from build123d import *

# Parameters (mm, degrees)
SKETCH1_R           = 3.29
BOSS_EXTRUDE1_DEPTH = 22
SKETCH2_W           = 24
SKETCH2_H           = 11
BOSS_EXTRUDE2_DEPTH = 3
SKETCH3_W           = 12
SKETCH3_H           = 25
CUT_EXTRUDE1_DEPTH  = 20.25


with BuildPart() as part:
    # Sketch1 → Boss-Extrude1 (new body)
    with BuildSketch(Plane(origin=(0, 0, 0), x_dir=(1, 0, 0), z_dir=(0, 1, 0))):
        Polygon((24, -29), (-24, -29), (-31, -21.49418526), (-32, 21.49418526), (-25, 29), (25, 29), (32, 21.49418526), (31, -21.49418526), align=None)
        with Locations(Location((-26.933648737, -2.8, 0), (0, 0, 270))):
            Circle(SKETCH1_R, mode=Mode.SUBTRACT)
        with Locations(Location((26.933648737, -2.8, 0), (0, 0, 270))):
            Circle(SKETCH1_R, mode=Mode.SUBTRACT)
    extrude(amount=BOSS_EXTRUDE1_DEPTH)

    # Sketch2 → Boss-Extrude2 (add)
    with BuildSketch(Plane.XY.offset(29)):
        with Locations((0, 5.5)):
            Rectangle(SKETCH2_W, SKETCH2_H)
    extrude(amount=BOSS_EXTRUDE2_DEPTH)

    # Sketch3 → Cut-Extrude1 (cut)
    with BuildSketch(Plane(origin=(0, 22, 0), x_dir=(1, 0, 0), z_dir=(0, 1, 0))):
        with Locations((-25.783797684, -0.3)):
            Rectangle(SKETCH3_W, SKETCH3_H)
        with Locations((25.783797684, -0.3)):
            Rectangle(SKETCH3_W, SKETCH3_H)
    extrude(amount=-CUT_EXTRUDE1_DEPTH, mode=Mode.SUBTRACT)


solid = part.part
For this review, take the finished solid that the model builds, in its own axes (mm). A direction names the side the tool comes from. Round coordinates to 2 decimals unless told otherwise and drop trailing zeros. Write each loop counter-clockwise with the first axis right and the second up, starting at its lowest first coordinate (ties: lowest second). Pieces come first, ordered by that corner, then holes. Notation, with made-up numbers: M 50,3.5 L 86,3.5 A25 cw 86,29.5 Z; hole C -12.5,47 d4. An arc over 180 degrees is marked long. Write item = value, one per line. Start each with the question number.
(1) We need section B-B (x = -21). Give the boundary of the cut face in (y, z).
(2) We need section C-C (z = 2.8). Give the boundary of the cut face in (x, y).
(3) The part is to be moulded in two halves that separate along Z. For faces 4 (the face through (0, 11, -29)), 5 (the face through (-24.5, 1.75, 0.1)), 6 (the face through (0, 6, 32)), 7 (the face through (0, 11, 30)), say which applies: +Z half, -Z half, draft (parallel to the pull), parting line (faces both ways), or undercut.
(4) For line 1 along X through (y, z) = (0.9, 2.8); line 2 along Z through (x, y) = (0.5, 19); line 3 along X through (y, z) = (20.5, 5), list the stretches that pass through material, from the lowest coordinate up.
(5) We need section A-A (y = 8.5). Give the boundary of the cut face in (x, z).
(6) For faces 1 (the face through (-26, 12, -12.2)), 2 (the face through (26, 12, -12.2)), 3 (the face through (12, 5, 30)), list the 3-axis set-ups (+Z, -Z, +X, -X, +Y, -Y) from which the entire face can be reached by the end or side of a thin tool; tool diameter is ignored.
(7) Clearance check with flat-ended pins moving along their axes: pin 1 Ø4 at (y, z) = (13, 11.5) entering from -X; pin 2 Ø8 at (x, y) = (20.5, 14) entering from +Z; pin 3 Ø1.5 at (y, z) = (9, 1.5) entering from -X. State where each tip first meets the part, or that it passes through.
(8) We need section D-D (x = -6). Give the boundary of the cut face in (y, z).
Results found:
q1.outline = M 0,-29 L 22,-29 L 22,-12.2 L 1.75,-12.2 L 1.75,12.8 L 22,12.8 L 22,29 L 0,29 Z
q2.outline = M -31.43,0 L -30.22,0 L -30.22,1.75 L -31.43,1.75 Z; M -23.64,0 L 23.64,0 L 23.64,1.75 L 19.78,1.75 L 19.78,22 L -19.78,22 L -19.78,1.75 L -23.64,1.75 Z; M 30.22,0 L 31.43,0 L 31.43,1.75 L 30.22,1.75 Z
q3.face_4 = -Z half
q3.face_5 = undercut
q3.face_6 = +Z half
q3.face_7 = draft
q4.line_1 = -31.43 to -30.22, -23.64 to 23.64, 30.22 to 31.43
q4.line_2 = -29 to 29
q4.line_3 = -19.78 to 19.78
q5.outline = M -32,-21.49 L -25,-29 L 25,-29 L 32,-21.49 L 31.78,-12.2 L 19.78,-12.2 L 19.78,12.8 L 31.2,12.8 L 31,21.49 L 24,29 L 12,29 L 12,32 L -12,32 L -12,29 L -24,29 L -31,21.49 L -31.2,12.8 L -19.78,12.8 L -19.78,-12.2 L -31.78,-12.2 Z
q6.face_1 = -X, +Y
q6.face_2 = +X, +Y
q6.face_3 = +Z, +X, +Y, -Y
q7.pin_1 = -31.2
q7.pin_2 = 29
q7.pin_3 = -19.78
q8.outline = M 0,-29 L 22,-29 L 22,29 L 11,29 L 11,32 L 0,32 Z
